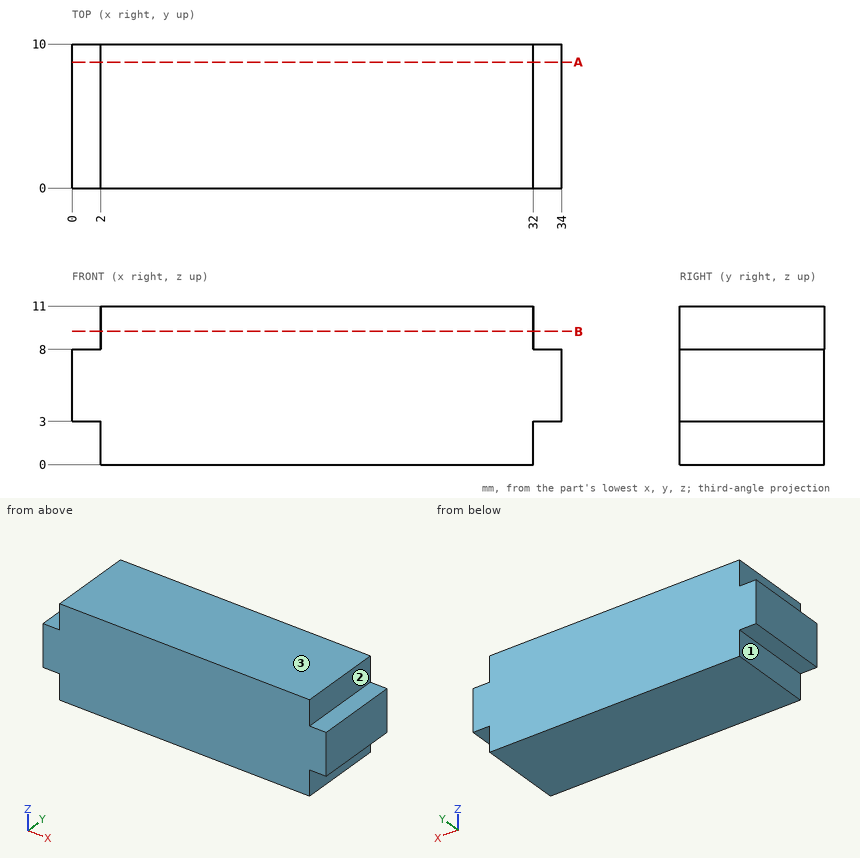
Could you check a few things on this drawing? It's one solid part, dimensions in mm from its lowest x, y, z. A direction names the side the tool comes from. Give positions to 0.01 mm unless a question says otherwise; leave off trailing zeros. Loops run counter-clockwise (first coordinate to the right, second up) from the corner with the lowest first, then second, coordinate; pieces in that order, holes last. Notation, with made-up numbers: M 61,-19 L 103,-19 A16 cw 103,-9 Z; hole C 72,-40 d3. An arc over 180 degrees is marked long. One line per question, with ' | ' between items. Start each with the question number.
Q1. If we section it at B-B (z = 9.25): Please give me the cut outline in (x, y), plus the area to 3 significant figures.
Q2. If I drill on line 1 (X direction, y = 7, z = 9.5), over which ranges is the centre line in solid material (lowest first)? Write a range as from..to.
Q3. For the marked faces 1, 2 and 3, which set-ups out of +Z, -Z, +X, -X, +Y, -Y let a thin tool reach every point of the face, with its end or its side?
Q4. For pin 1 Ø0.9 at (y, z) = (7, 10) entering from -X; pin 2 Ø2.5 at (y, z) = (7.5, 10) entering from +X; pin 3 Ø0.6 at (x, y) = (0.5, 4) entering from -Z, each with a flat end and sliding along its axis, tell me the tip position at first contact or that it passes through.
Q5. If we section it at A-A (y = 8.75): Please give me the cut outline in (x, z).
Computed:
1) outline: M 2,0 L 32,0 L 32,10 L 2,10 Z | area: 300 mm²
2) line 1: x = 2..32
3) face 1: -Z, -X, +Y, -Y | face 2: +Z, +X, +Y, -Y | face 3: +Z, +X, -X, +Y, -Y
4) pin 1: stops at x = 2 | pin 2: stops at x = 32 | pin 3: stops at z = 3
5) outline: M 0,3 L 2,3 L 2,0 L 32,0 L 32,3 L 34,3 L 34,8 L 32,8 L 32,11 L 2,11 L 2,8 L 0,8 Z
